```python
from build123d import *

# Parameters (mm, degrees)
ESQUISSE1_R             = 52.5
ESQUISSE1_R_2           = 2.05
ESQUISSE1_R_3           = 1.3
ESQUISSE1_R_4           = 10
BOSS_EXTRU_2_DEPTH      = 5
ESQUISSE2_R             = 52.5
BOSS_EXTRU_3_DEPTH      = 37.5
ENL_V_START             = -4
ESQUISSE3_R             = 3.35
ENL_V_MAT_EXTRU_1_DEPTH = 82.549693161
ESQUISSE5_R             = 1.55
ENL_V_MAT_EXTRU_3_DEPTH = 86.549693161
ESQUISSE6_R             = 3.75
ENL_V_MAT_EXTRU_4_DEPTH = 3
ESQUISSE7_W             = 25
ESQUISSE7_H             = 37.5
ENL_V_MAT_EXTRU_5_DEPTH = 86.549693161
BOSS_EXTRU_5_DEPTH      = 5
BOSS_EXTRU_9_DEPTH      = 37.5
CONG_1_R                = 10


with BuildPart() as part:
    # Esquisse1 → Boss.-Extru.2 (new body)
    with BuildSketch(Plane(origin=(0, 0, 0), x_dir=(1, 0, 0), z_dir=(0, 1, 0))):
        with Locations(Location((0, 0, 0), (0, 0, 270))):
            Circle(ESQUISSE1_R)
        with Locations(Location((0, 40, 0), (0, 0, 270))):
            Circle(ESQUISSE1_R_2, mode=Mode.SUBTRACT)
        with Locations(Location((40, 0, 0), (0, 0, 270))):
            Circle(ESQUISSE1_R_2, mode=Mode.SUBTRACT)
        with Locations(Location((0, -40, 0), (0, 0, 270))):
            Circle(ESQUISSE1_R_2, mode=Mode.SUBTRACT)
        with Locations(Location((-40, 0, 0), (0, 0, 270))):
            Circle(ESQUISSE1_R_2, mode=Mode.SUBTRACT)
        with Locations(Location((28, 28, 0), (0, 0, 270))):
            Circle(ESQUISSE1_R_3, mode=Mode.SUBTRACT)
        with Locations(Location((20, -42, 0), (0, 0, 270))):
            Circle(ESQUISSE1_R_3, mode=Mode.SUBTRACT)
        with Locations(Location((-20, -42, 0), (0, 0, 90))):
            Circle(ESQUISSE1_R_3, mode=Mode.SUBTRACT)
        with Locations(Location((-28, 28, 0), (0, 0, 90))):
            Circle(ESQUISSE1_R_3, mode=Mode.SUBTRACT)
        with Locations(Location((0, 0, 0), (0, 0, 270))):
            Circle(ESQUISSE1_R_4, mode=Mode.SUBTRACT)
    extrude(amount=BOSS_EXTRU_2_DEPTH)

    # Esquisse2 → Boss.-Extru.3 (add)
    with BuildSketch(Plane(origin=(0, 5, 0), x_dir=(1, 0, 0), z_dir=(0, 1, 0))):
        with Locations(Location((0, 0, 0), (0, 0, 270))):
            Circle(ESQUISSE2_R)
        with BuildLine():
            ThreePointArc((-4.5, 47.5), (0, 43), (4.5, 47.5))
            Line((4.5, 47.5), (4.5, 48.062459363))
            ThreePointArc((4.5, 48.062459363), (5.183960957, 49.568461102), (6.768041237, 50.04441645))
            ThreePointArc((6.768041237, 50.04441645), (43.734282891, 25.25), (46.723756582, -19.16091258))
            ThreePointArc((46.723756582, -19.16091258), (45.519527019, -20.29478867), (43.873310777, -20.134115364))
            Line((43.873310777, -20.134115364), (43.38620668, -19.852885683))
            ThreePointArc((43.38620668, -19.852885683), (37.239092363, -21.5), (38.88620668, -27.647114317))
            Line((38.88620668, -27.647114317), (39.373310777, -27.928343998))
            ThreePointArc((39.373310777, -27.928343998), (40.335566062, -29.273672432), (39.955715345, -30.88350387))
            ThreePointArc((39.955715345, -30.88350387), (0, -50.5), (-39.955715345, -30.88350387))
            ThreePointArc((-39.955715345, -30.88350387), (-40.335566062, -29.273672432), (-39.373310777, -27.928343998))
            Line((-39.373310777, -27.928343998), (-38.88620668, -27.647114317))
            ThreePointArc((-38.88620668, -27.647114317), (-37.239092363, -21.5), (-43.38620668, -19.852885683))
            Line((-43.38620668, -19.852885683), (-43.873310777, -20.134115364))
            ThreePointArc((-43.873310777, -20.134115364), (-45.519527019, -20.29478867), (-46.723756582, -19.16091258))
            ThreePointArc((-46.723756582, -19.16091258), (-43.734282891, 25.25), (-6.768041237, 50.04441645))
            ThreePointArc((-6.768041237, 50.04441645), (-5.183960957, 49.568461102), (-4.5, 48.062459363))
            Line((-4.5, 48.062459363), (-4.5, 47.5))
        make_face(mode=Mode.SUBTRACT)
    extrude(amount=BOSS_EXTRU_3_DEPTH)

    # Esquisse3 → Enlèv. mat.-Extru.1 (cut, through all)
    with BuildSketch(Plane(origin=(0, 42.5, 0), x_dir=(1, 0, 0), z_dir=(0, 1, 0)).offset(ENL_V_START)):
        with Locations(Location((0, 47.5, 0), (0, 0, 270))):
            Circle(ESQUISSE3_R)
        with Locations(Location((41.13620668, -23.75, 0), (0, 0, 270))):
            Circle(ESQUISSE3_R)
        with Locations(Location((-41.13620668, -23.75, 0), (0, 0, 270))):
            Circle(ESQUISSE3_R)
    extrude(amount=-ENL_V_MAT_EXTRU_1_DEPTH, mode=Mode.SUBTRACT)

    # Esquisse5 → Enlèv. mat.-Extru.3 (cut, through all)
    with BuildSketch(Plane(origin=(0, 42.5, 0), x_dir=(1, 0, 0), z_dir=(0, 1, 0))):
        with Locations(Location((-41.13620668, -23.75, 0), (0, 0, 270))):
            Circle(ESQUISSE5_R)
        with Locations(Location((41.13620668, -23.75, 0), (0, 0, 270))):
            Circle(ESQUISSE5_R)
        with Locations(Location((0, 47.5, 0), (0, 0, 270))):
            Circle(ESQUISSE5_R)
    extrude(amount=-ENL_V_MAT_EXTRU_3_DEPTH, mode=Mode.SUBTRACT)

    # Esquisse6 → Enlèv. mat.-Extru.4 (cut)
    with BuildSketch(Plane.XZ):
        with Locations(Location((-20, 42, 0), (0, 0, 270))):
            Circle(ESQUISSE6_R)
        with Locations(Location((20, 42, 0), (0, 0, 270))):
            Circle(ESQUISSE6_R)
        with Locations(Location((-28, -28, 0), (0, 0, 270))):
            Circle(ESQUISSE6_R)
        with Locations(Location((28, -28, 0), (0, 0, 270))):
            Circle(ESQUISSE6_R)
    extrude(amount=-ENL_V_MAT_EXTRU_4_DEPTH, mode=Mode.SUBTRACT)

    # Esquisse7 → Enlèv. mat.-Extru.5 (cut, through all)
    with BuildSketch(Plane.XY):
        with Locations((-12.5, 23.75)):
            Rectangle(ESQUISSE7_W, ESQUISSE7_H)
        with Locations((12.5, 23.75)):
            Rectangle(ESQUISSE7_W, ESQUISSE7_H)
    extrude(amount=ENL_V_MAT_EXTRU_5_DEPTH, mode=Mode.SUBTRACT)

    # Esquisse8 → Boss.-Extru.5 (add)
    with BuildSketch(Plane(origin=(0, 0, 0), x_dir=(1, 0, 0), z_dir=(0, 1, 0))):
        with BuildLine():
            ThreePointArc((-25, -46.165463282), (0, -65.749037603), (25, -46.165463282))
            ThreePointArc((25, -46.165463282), (0, -52.5), (-25, -46.165463282))
        make_face()
    extrude(amount=BOSS_EXTRU_5_DEPTH)

    # Esquisse11 → Boss.-Extru.9 (add)
    with BuildSketch(Plane(origin=(0, 5, 0), x_dir=(1, 0, 0), z_dir=(0, 1, 0))):
        with BuildLine():
            Line((0, -65.749037603), (0, -63.749037603))
            ThreePointArc((0, -63.749037603), (-14.989303659, -58.421117308), (-23.2531293, -44.827915162))
            ThreePointArc((-23.2531293, -44.827915162), (-24.131242464, -44.361392416), (-25, -43.877670859))
            Line((-25, -43.877670859), (-25, -46.165463282))
            ThreePointArc((-25, -46.165463282), (-15.878573481, -60.270269896), (0, -65.749037603))
        make_face()
        with BuildLine():
            ThreePointArc((23.2531293, -44.827915162), (14.989303659, -58.421117308), (0, -63.749037603))
            Line((0, -63.749037603), (0, -65.749037603))
            ThreePointArc((0, -65.749037603), (15.878573481, -60.270269896), (25, -46.165463282))
            Line((25, -46.165463282), (25, -43.877670859))
            ThreePointArc((25, -43.877670859), (24.131242464, -44.361392416), (23.2531293, -44.827915162))
        make_face()
    extrude(amount=BOSS_EXTRU_9_DEPTH)

    # Congé1
    cong_1_edges = [part.edges().sort_by_distance(p)[0] for p in [
        (25, 21.25, 46.165463282),
        (-25, 21.25, 46.165463282),
        (23.2531293, 23.75, 44.827915162),
        (-23.2531293, 23.75, 44.827915162),
    ]]
    fillet(cong_1_edges, radius=CONG_1_R)


solid = part.part
```
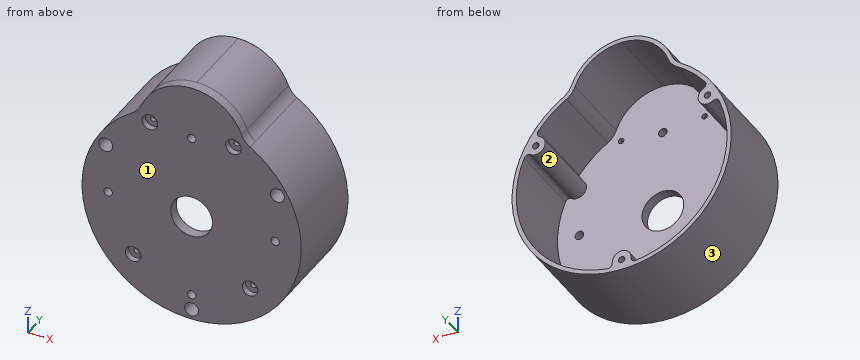
For this review, take the finished solid that the model builds, in its own axes (mm). Face numbers are marked on the shaded views. Coordinates: 2 decimals unless noted, no trailing zeros. Write each loop counter-clockwise with the first axis right and the second up, starting at its lowest first coordinate (ties: lowest second). Pieces come first, ordered by that corner, then holes.
(1) The part is to be moulded in two halves that separate along X. For the marked faces 1, 2 and 3, say which applies: +X half, -X half, draft (parallel to the pull), parting line (faces both ways), or undercut.
(2) Wall thickness on probe 1 along X at (y, z) = (2.8, 0); probe 2 along X at (y, z) = (2.55, 40); probe 3 along X at (y, z) = (28, 1.5): over which ranges is each line inside the solid? List them lowest first.
(3) Add section A-A on z = 0. Give the boundary of the cut face in (x, y), then the cut area to 3 significant figures.
(4) Add section B-B on x = -8.5. Give the boundary of the cut face in (y, z).
(5) Add section D-D on y = 36. Count the separate pieces of the cut face and the enclosed holes in it, then the cut area to 3 significant figures.
(6) For pin 1 Ø16 at (x, z) = (0, 0) entering from -Y; pin 2 Ø2 at (x, y) = (11, 34.5) entering from -Z; pin 3 Ø8 at (y, z) = (18, -6) entering from +X; pin 4 Ø1.5 at (y, z) = (31, 12.5) entering from +X, all flat-tipped, find the tip position at first contact; note any pin that passes through.
(7) Add section C-C on z = 36. Give the boundary of the cut face in (x, y).
Answer sheet:
1. face 1: draft
1. face 2: undercut
1. face 3: parting line
2. probe 1: x = -52.5 to -42.05, -37.95 to -10, 10 to 37.95, 42.05 to 52.5
2. probe 2: x = -34 to -23.17, -16.83 to -2.05, 2.05 to 16.83, 23.17 to 34
2. probe 3: x = -52.48 to -50.48, 50.48 to 52.48
3. outline: (-52.5, 0) - (-42.05, 0) - (-42.05, 5) - (-50.5, 5) - (-50.5, 42.5) - (-52.5, 42.5) - close; (-37.95, 0) - (-10, 0) - (-10, 5) - (-37.95, 5) - close; (10, 0) - (37.95, 0) - (37.95, 5) - (10, 5) - close; (42.05, 0) - (52.5, 0) - (52.5, 42.5) - (50.5, 42.5) - (50.5, 5) - (42.05, 5) - close
3. area: 534 mm2
4. outline: (0, -51.81) - (42.5, -51.81) - (42.5, -49.78) - (5, -49.78) - (5, -5.27) - (0, -5.27) - close; (0, 5.27) - (5, 5.27) - (5, 62.18) - (42.5, 62.18) - (42.5, 64.31) - (0, 64.31) - close
5. separate pieces: 1
5. enclosed holes: 4
5. area: 755 mm2
6. pin 1: passes through
6. pin 2: stops at z = -51.54
6. pin 3: stops at x = 52.46
6. pin 4: stops at x = 51.17
7. outline: (-38.21, 0) - (38.21, 0) - (38.21, 42.5) - (35.42, 42.5) - (35.42, 5) - (-35.42, 5) - (-35.42, 42.5) - (-38.21, 42.5) - close
